Drawing for the job (mm, zero at the part's lowest x, y, z). Coordinates: 2 decimals unless noted, no trailing zeros. Write each loop counter-clockwise with the first axis right and the second up, starting at its lowest first coordinate (ties: lowest second). Pieces come first, ordered by that corner, then holes. Notation, with made-up numbers: (-13.5, -4.75) - (-0.5, -4.75) arc R31 ccw to (-0.5, 21.25) - close; hole circle Ø6 at (7.5, 64.5). An arc over 180 degrees is marked (long way). Write each question's results on one line, items separated by ' | '.
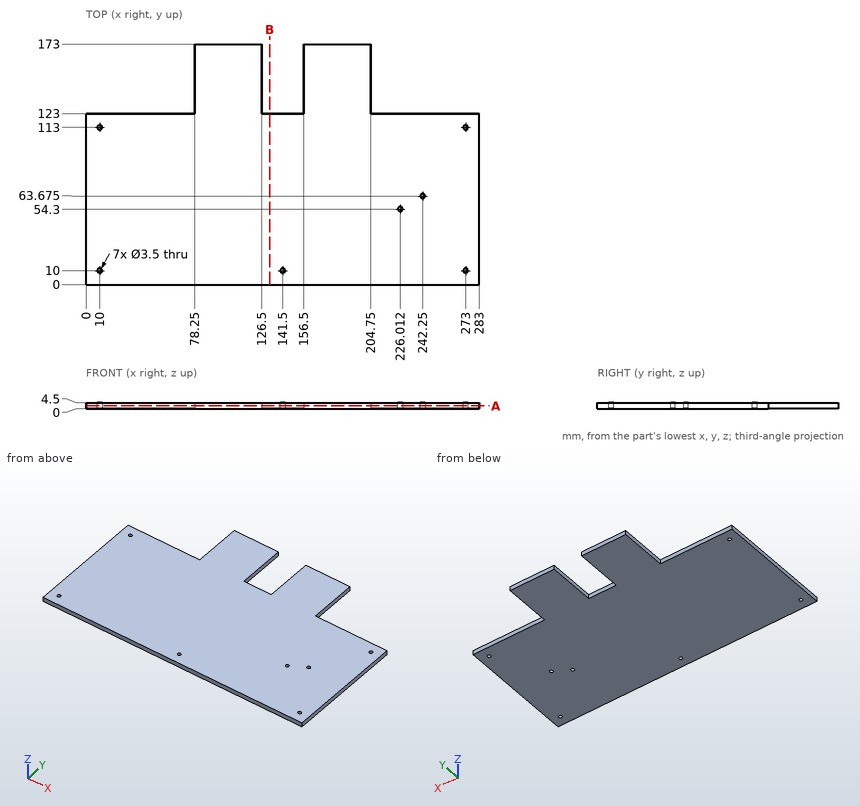
(1) Wall check: line 1 (Y direction, x = 10, z = 1.3); line 2 (X direction, y = 10, z = 0.95); line 3 (X direction, y = 54.3, z = 2.7). Give the ranges that are in metal, low to high. Write a range as from..to.
Return value:
line 1: y = 0..8.25, 11.75..111.25, 114.75..123 | line 2: x = 0..8.25, 11.75..139.75, 143.25..271.25, 274.75..283 | line 3: x = 0..224.26, 227.76..283
(2) Saw through at A-A on z = 2.1. Write the cut outline in (x, y) (3 decimals).
Return value:
outline: (0, 0) - (283, 0) - (283, 123) - (204.75, 123) - (204.75, 173) - (156.5, 173) - (156.5, 123) - (126.5, 123) - (126.5, 173) - (78.25, 173) - (78.25, 123) - (0, 123) - close; hole circle Ø3.5 at (10, 10); hole circle Ø3.5 at (10, 113); hole circle Ø3.5 at (141.5, 10); hole circle Ø3.5 at (226.012, 54.3); hole circle Ø3.5 at (242.25, 63.675); hole circle Ø3.5 at (273, 10); hole circle Ø3.5 at (273, 113)
(3) Flat gauge pins, fed straight in: P1, Ø2, axis at y = 136.5, z = 3.5, coming from the +X side; P2, Ø1.3, axis at y = 136.5, z = 3, coming from the -X side. Where does each tip first touch, or does it go through?
Return value:
P1: stops at x = 204.75 | P2: stops at x = 78.25
(4) Saw through at B-B on x = 132. Write the cut outline in (y, z), then the cut area to 4 significant figures.
Return value:
outline: (0, 0) - (123, 0) - (123, 4.5) - (0, 4.5) - close | area: 553.5 mm^2
